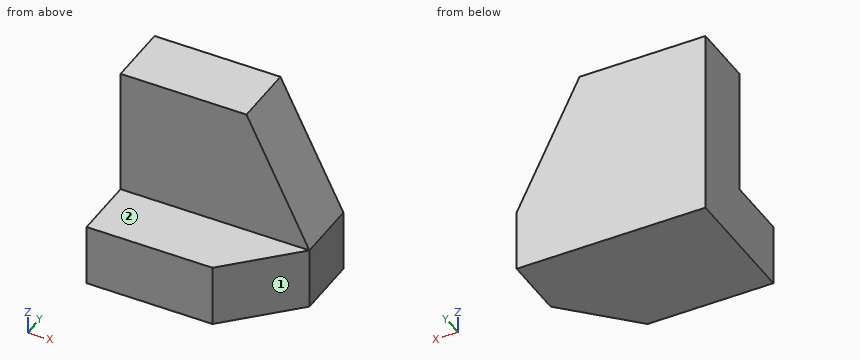
from build123d import *

# Parameters (mm, degrees)
F1_DEPTH = 38.1
F3_DEPTH = 25.4
F5_DEPTH = 25.4


with BuildPart() as f1:
    # F0 (on Right) → F1 (new body)
    with BuildSketch(Plane.YZ):
        Polygon((12.7, 12.482905), (0, 12.482905), (0, 0), (25.4, 0), (25.4, 38.1), (12.7, 38.1), align=None)
    extrude(amount=F1_DEPTH)

    # F2 (on face) → F3 (cut)
    with BuildSketch(Plane.XZ.offset(-12.7)):
        Polygon((38.1, 38.1), (25.4, 38.1), (38.1, 12.482905), align=None)
    extrude(amount=-F3_DEPTH, mode=Mode.SUBTRACT)

    # F4 (on face) → F5 (cut)
    with BuildSketch(Plane.XY.offset(12.482905)):
        Polygon((38.1, 0), (38.1, 12.7), (25.4, 0), align=None)
    extrude(amount=-F5_DEPTH, mode=Mode.SUBTRACT)


solid = f1.part
Input: part model. Units: mm. Frame: model coordinates. Face numbers are marked on the shaded views. A direction names the side the tool comes from. Give positions to 0.01 mm unless a question says otherwise; leave off trailing zeros. Order: outer loops, then holes, each group sorted by start corner. A loop starts at its lowest first (then second) coordinate and runs counter-clockwise, first axis right, second up. Notation, with made-up numbers: (10.25, 0) - (29.25, 0) arc R33 ccw to (29.25, 30) - close; hole circle Ø1 at (70.25, -39.5). An arc over 180 degrees is marked (long way). Answer as a JSON object with one key per item and string values. Group by question number.
Q1. Cut plane B-B, the plane z = 7.5. Output: boundary loops of the cut face in (x, y), then the cut area to 3 significant figures.
Q2. Line query: probe 1 along Y at (x, z) = (16, 21); probe 2 along Z at (x, y) = (5, 5.75); probe 3 along X at (y, z) = (15.25, 24). Output: solid intervals per line, ascending.
Q3. Cut plane C-C, the plane y = 19. Output: boundary loops of the cut face in (x, z), then the cut area to 3 significant figures.
Q4. Cut plane D-D, the plane y = 2.25. Output: boundary loops of the cut face in (x, z).
Q5. Cut plane A-A, the plane x = 10.5. Output: boundary loops of the cut face in (y, z), then the cut area to 3 significant figures.
Q6. First-contact query: pin 1 Ø8 at (x, z) = (9, 21.5) entering from -Y; pin 2 Ø6 at (y, z) = (6, 12) entering from +X; pin 3 Ø1 at (x, y) = (8, 11.5) entering from +Z. Flat tips, straight axial feed; report the tip coordinate or a pass-through.
Q7. Set-up query: the marked faces 1 and 2. Return all of +Z, -Z, +X, -X, +Y, -Y with unobstructed straight access to the full face (end or side cutting, diameter ignored); none if empty.
Results:
{
 "1": {"outline": "(0, 0) - (25.4, 0) - (38.1, 12.7) - (38.1, 25.4) - (0, 25.4) - close", "area": "887 mm^2"},
 "2": {"probe 1": "12.7 to 25.4", "probe 2": "0 to 12.48", "probe 3": "0 to 32.39"},
 "3": {"outline": "(0, 0) - (38.1, 0) - (38.1, 12.48) - (25.4, 38.1) - (0, 38.1) - close", "area": "1,290 mm^2"},
 "4": {"outline": "(0, 0) - (27.65, 0) - (27.65, 12.48) - (0, 12.48) - close"},
 "5": {"outline": "(0, 0) - (25.4, 0) - (25.4, 38.1) - (12.7, 38.1) - (12.7, 12.48) - (0, 12.48) - close", "area": "642 mm^2"},
 "6": {"pin 1": "y = 12.7", "pin 2": "x = 34.4", "pin 3": "z = 12.48"},
 "7": {"face 1": "+Z, -Z, +X, -Y", "face 2": "+Z, +X, -X, -Y"}
}
